Input: part model. Units: mm. Frame: model coordinates. A direction names the side the tool comes from. Give positions to 0.01 mm unless a question says otherwise; leave off trailing zeros. Write each loop counter-clockwise with the first axis right and the second up, starting at its lowest first coordinate (ties: lowest second). Pieces come first, ordered by that corner, then holes. Notation, with made-up numbers: (76, 69.5) -> (84, 69.5) arc R17 ccw to (84, 98.5) -> close; hole circle Ø7 at (-13.75, 28.25). An arc over 180 degrees is marked (long way). Return JSON: item names as keys, results as strings. Group by question number.
Item 1: Set-up query: faces 1 (the face through (24.54, -14.96, 8.5)), 2 (the face through (-30, 0, 0)). Return all of +Z, -Z, +X, -X, +Y, -Y with unobstructed straight access to the full face (end or side cutting, diameter ignored); none if empty.
Item 2: Section A-A, the plane x = 7. Return loops of the section in (y, z), then the cut area to 3 significant figures.
Item 3: Pin query (flat end, axial travel): P1, Ø1.5, axis at x = -2, z = -9, coming from the -Y side. Return the tip coordinate at first contact, or that it passes through.
Item 4: Section D-D, the plane x = 15. Return loops of the section in (y, z).
Item 5: Line query: line 1 (Y direction, x = 19.5, z = -3.5); line 2 (X direction, y = -14.5, z = 2.5). Output: solid intervals per line, ascending. Write a range as [from, to].
Item 6: Section B-B, the plane y = -13.5. Return loops of the section in (x, z).
Item 7: Section C-C, the plane z = -14.5. Return loops of the section in (x, y).
from build123d import *

# Parameters (mm, degrees)
F0_W     = 60
F0_H     = 41
F1_DEPTH = 12.35
F2_R     = 10
F2_R_2   = 5
F3_DEPTH = 5.3


with BuildPart() as f1:
    # F0 (on Front) → F1 (new body, symmetric)
    with BuildSketch(Plane.XZ):
        Rectangle(F0_W, F0_H)
    extrude(amount=F1_DEPTH, both=True)

    # F2 (on face) → F3 (join)
    with BuildSketch(Plane.XZ.offset(12.35)):
        with Locations((15, 5.5)):
            Circle(F2_R)
        with Locations((-20, 5.5)):
            Circle(F2_R_2)
    extrude(amount=F3_DEPTH)


solid = f1.part
Answer below:
{
 "1": {"face 1": "-Y", "face 2": "+Z, -Z, -X, +Y, -Y"},
 "2": {"outline": "(-17.65, -0.5) -> (-12.35, -0.5) -> (-12.35, -20.5) -> (12.35, -20.5) -> (12.35, 20.5) -> (-12.35, 20.5) -> (-12.35, 11.5) -> (-17.65, 11.5) -> close", "area": "1,080 mm2"},
 "3": {"P1": "stops at y = -12.35"},
 "4": {"outline": "(-17.65, -4.5) -> (-12.35, -4.5) -> (-12.35, -20.5) -> (12.35, -20.5) -> (12.35, 20.5) -> (-12.35, 20.5) -> (-12.35, 15.5) -> (-17.65, 15.5) -> close"},
 "5": {"line 1": "y = [-12.35, 12.35]", "line 2": "x = [-24, -16], [5.46, 24.54]"},
 "6": {"outline": "circle Ø10 at (-20, 5.5); circle Ø20 at (15, 5.5)"},
 "7": {"outline": "(-30, -12.35) -> (30, -12.35) -> (30, 12.35) -> (-30, 12.35) -> close"}
}
